The figure shows three views and two pictorial views of one solid part (mm, origin at its lowest corner). Answer the questions. Give positions to 0.01 mm unless a question says otherwise; leave off trailing zeros. One line per question, with ' | ' between items. Start each with the question number.
1. Find the intervals of material crossed by L1, parallel to Y at x = 3.5, z = 32.45 (1 decimal); L2, parallel to Y at x = 4, z = 19.4 (1 decimal); L3, parallel to Y at x = 5.75, z = 34.5 (1 decimal), in increasing order. Write a range as from..to.
2. The mould has two halves that part along X. Classify the marked faces 1, 2 and 3: +X half, -X half, draft (parallel to the pull), parting line (faces both ways), or undercut.
3. Given P1, Ø1, axis at x = 3.5, z = 5.5, coming from the +Y side, flat-ended and moving along its own axis, determine where the tip first touches the part or whether it passes through.
4. A cutting plane is placed at B-B (x = 1). State how many separate pieces and enclosed holes the cut face has, then the cut area to 3 significant figures.
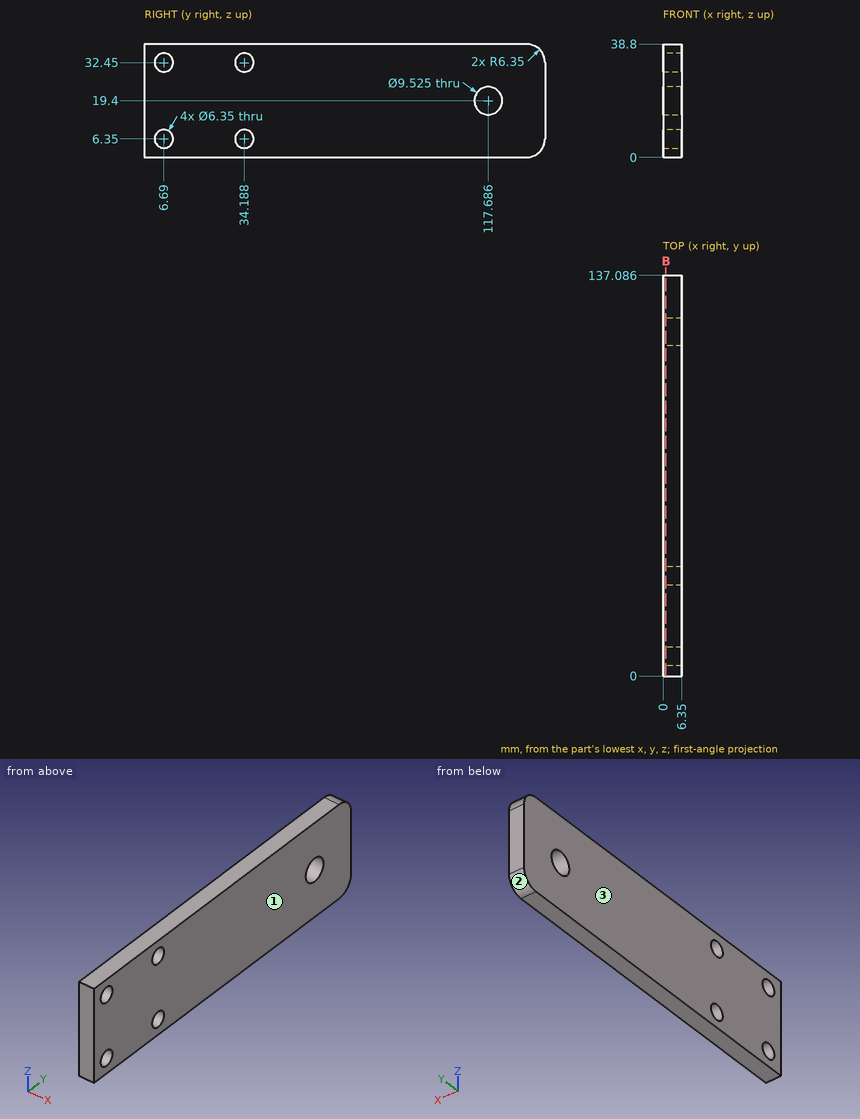
Determined:
1) L1: 0..3.5, 9.9..31, 37.4..137.1 | L2: 0..112.9, 122.4..137.1 | L3: 0..4.3, 9.1..31.8, 36.6..136.7
2) face 1: +X half | face 2: draft | face 3: -X half
3) P1: y = 137.08
4) separate pieces: 1 | enclosed holes: 5 | area: 5,100 mm2
